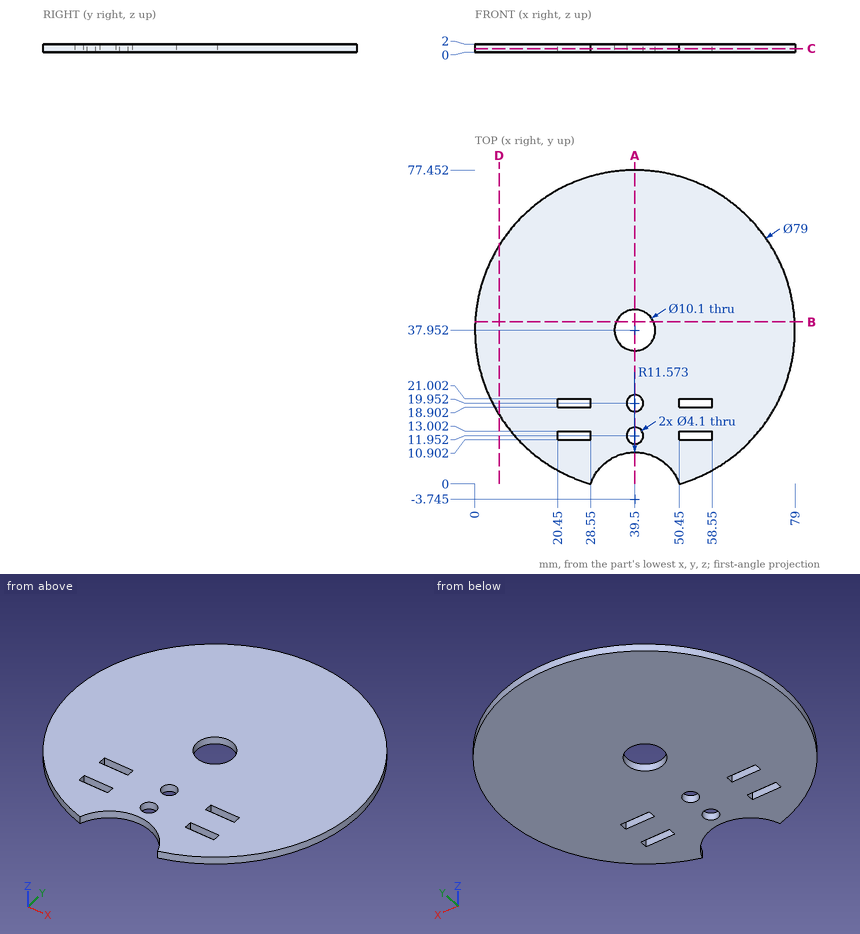
Drawing for the job (mm, zero at the part's lowest x, y, z). Round coordinates to 2 decimals unless told otherwise and drop trailing zeros. Write each loop counter-clockwise with the first axis right and the second up, starting at its lowest first coordinate (ties: lowest second). Pieces come first, ordered by that corner, then holes. Notation, with made-up numbers: (0.5, 31) - (7.5, 31) arc R13 cw to (7.5, 43) - close; hole circle Ø3 at (53.5, 55). An arc over 180 degrees is marked (long way). Return JSON: item names as keys, results as strings. Group by question number.
Item 1: Band-saw the part on A-A on x = 39.5. List the corners of the cut face in (y, z), plus the area to 3 significant figures.
Item 2: Flat gauge pins, fed straight in: pin 1 Ø1 at (x, z) = (56, 0.5) entering from -Y; pin 2 Ø0.6 at (x, z) = (55, 1.5) entering from +Y; pin 3 Ø0.6 at (y, z) = (20, 1) entering from -X. Where does each tip first touch, or does it go through?
Item 3: Band-saw the part on C-C on z = 0.85. State how many separate pieces and enclosed holes the cut face has, plus the area to 3 significant figures.
Item 4: Band-saw the part on B-B on y = 40. List the corners of the cut face in (x, z), plus the area to 3 significant figures.
Item 5: Band-saw the part on D-D on x = 6. List the corners of the cut face in (y, z).
Item 6: Probe probe 1 along Y at (x, z) = (39.5, 1.65); probe 2 along Y at (x, z) = (54, 0.8) (1 decimal); probe 3 along Y at (x, z) = (26.5, 0.65). List the from-to ranges inside material, lowest first.
Resolved:
{
 "1": {"outline": "(7.83, 0) - (9.9, 0) - (9.9, 2) - (7.83, 2) - close; (14, 0) - (17.9, 0) - (17.9, 2) - (14, 2) - close; (22, 0) - (32.9, 0) - (32.9, 2) - (22, 2) - close; (43, 0) - (77.45, 0) - (77.45, 2) - (43, 2) - close", "area": "103 mm²"},
 "2": {"pin 1": "stops at y = 1.84", "pin 2": "stops at y = 74.41", "pin 3": "stops at x = 4.16"},
 "3": {"separate pieces": "1", "enclosed holes": "7", "area": "4,580 mm²"},
 "4": {"outline": "(0.05, 0) - (34.88, 0) - (34.88, 2) - (0.05, 2) - close; (44.12, 0) - (78.95, 0) - (78.95, 2) - (44.12, 2) - close", "area": "139 mm²"},
 "5": {"outline": "(17.02, 0) - (58.88, 0) - (58.88, 2) - (17.02, 2) - close"},
 "6": {"probe 1": "y = 7.83 to 9.9, 14 to 17.9, 22 to 32.9, 43 to 77.45", "probe 2": "y = 1.2 to 10.9, 13 to 18.9, 21 to 74.7", "probe 3": "y = 0.65 to 10.9, 13 to 18.9, 21 to 75.25"}
}
